from build123d import *

# Parameters (mm, degrees)
SKETCH1_W                    = 49.788
SKETCH1_H                    = 49.788
BOSS_EXTRUDE1_DEPTH          = 3
SKETCH1_3_W                  = 55.788
SKETCH1_3_H                  = 55.788
SKETCH1_3_W_2                = 49.788
SKETCH1_3_H_2                = 49.788
BOSS_EXTRUDE2_DEPTH          = 118
SKETCH2_W                    = 49.788
SKETCH2_H                    = 3
SKETCH2_W_2                  = 43.788
SKETCH2_H_2                  = 38.949
SKETCH2_H_3                  = 26.974
SKETCH2_H_4                  = 16.077
CUT_EXTRUDE1_DEPTH           = 3
FILLET1_R                    = 2
SKETCH3_W                    = 43.788
SKETCH3_H                    = 106
CUT_EXTRUDE2_DEPTH           = 56
FILLET2_R                    = 2
SKETCH4_W                    = 5
SKETCH4_H                    = 3
CUT_EXTRUDE3_DEPTH           = 3
CSK_FOR_M4_SFHCS1_AT_2_COUNT = 2
CSK_FOR_M4_SFHCS1_AT_2_PITCH = 46.834641181
CSK_FOR_M4_SFHCS1_AT_3_COUNT = 2
CSK_FOR_M4_SFHCS1_AT_3_PITCH = 46.834641181
FILLET3_R                    = 1


with BuildPart() as part:
    # Sketch1 → Boss-Extrude1 (new body)
    with BuildSketch(Plane(origin=(0, 0, 0), x_dir=(1, 0, 0), z_dir=(0, 1, 0))):
        Rectangle(SKETCH1_W, SKETCH1_H)
    extrude(amount=BOSS_EXTRUDE1_DEPTH)

    # Sketch1_3 → Boss-Extrude2 (add)
    with BuildSketch(Plane(origin=(0, 0, 0), x_dir=(1, 0, 0), z_dir=(0, 1, 0))):
        Rectangle(SKETCH1_3_W, SKETCH1_3_H)
        Rectangle(SKETCH1_3_W_2, SKETCH1_3_H_2, mode=Mode.SUBTRACT)
    extrude(amount=BOSS_EXTRUDE2_DEPTH)

    # Sketch2 → Cut-Extrude1 (cut)
    with BuildSketch(Plane(origin=(27.894, 0, 0), x_dir=(0, 0, -1), z_dir=(1, 0, 0))):
        with Locations((0, 90.423)):
            Rectangle(SKETCH2_W, SKETCH2_H)
        with Locations((0, 38.474)):
            Rectangle(SKETCH2_W, SKETCH2_H)
        with Locations((0, 64.4485)):
            Rectangle(SKETCH2_W_2, SKETCH2_H_2)
        with Locations((0, 18.487)):
            Rectangle(SKETCH2_W_2, SKETCH2_H_3)
        with Locations((0, 104.9615)):
            Rectangle(SKETCH2_W_2, SKETCH2_H_4)
    extrude(amount=-CUT_EXTRUDE1_DEPTH, mode=Mode.SUBTRACT)

    # Fillet1
    fillet1_edges = [part.edges().sort_by_distance(p)[0] for p in [
        (26.394, 96.923, 21.894),
        (26.394, 113, 21.894),
        (26.394, 113, -21.894),
        (26.394, 96.923, -21.894),
        (26.394, 44.974, 21.894),
        (26.394, 83.923, 21.894),
        (26.394, 83.923, -21.894),
        (26.394, 44.974, -21.894),
        (26.394, 5, 21.894),
        (26.394, 31.974, 21.894),
        (26.394, 31.974, -21.894),
        (26.394, 5, -21.894),
    ]]
    fillet(fillet1_edges, radius=FILLET1_R)

    # Sketch3 → Cut-Extrude2 (cut)
    with BuildSketch(Plane(origin=(0, 0, -27.894), x_dir=(-1, 0, 0), z_dir=(0, 0, -1))):
        with Locations((0, 59)):
            Rectangle(SKETCH3_W, SKETCH3_H)
    extrude(amount=-CUT_EXTRUDE2_DEPTH, mode=Mode.SUBTRACT)

    # Fillet2
    fillet2_edges = [part.edges().sort_by_distance(p)[0] for p in [
        (21.894, 6, -26.394),
        (21.894, 6, 26.394),
        (21.894, 112, -26.394),
        (21.894, 112, 26.394),
        (-21.894, 112, -26.394),
        (-21.894, 112, 26.394),
        (-21.894, 6, -26.394),
        (-21.894, 6, 26.394),
    ]]
    fillet(fillet2_edges, radius=FILLET2_R)

    # Sketch4 → Cut-Extrude3 (cut)
    with BuildSketch(Plane.ZY.offset(27.894)):
        with Locations((0, 90.423)):
            Rectangle(SKETCH4_W, SKETCH4_H)
        with Locations((0, 40.474)):
            Rectangle(SKETCH4_W, SKETCH4_H)
    extrude(amount=-CUT_EXTRUDE3_DEPTH, mode=Mode.SUBTRACT)

    # Sketch7 → CSK for M4 SFHCS1 (revolve, cut)
    with BuildSketch(Plane(origin=(-24.894, 65.538290214, -0.216772751), x_dir=(0, 0, -1), z_dir=(0, 1, 0))):
        Polygon((0, 0), (0, 3), (2.25, 3), (2.25, 2.23), (4.48, 0), align=None)
    csk_for_m4_sfhcs1 = revolve(axis=Axis((-18.544, 65.538290214, -0.216772751), (-1, 0, 0)), mode=Mode.SUBTRACT)

    # CSK for M4 SFHCS1 at 2: CSK for M4 SFHCS1 ×2
    with Locations(*[Vector(0, -0.999997358, -0.002298525) * (i * CSK_FOR_M4_SFHCS1_AT_2_PITCH) for i in range(1, CSK_FOR_M4_SFHCS1_AT_2_COUNT)]):
        add(csk_for_m4_sfhcs1, mode=Mode.SUBTRACT)

    # CSK for M4 SFHCS1 at 3: CSK for M4 SFHCS1 ×2
    with Locations(*[Vector(0, -0.999997358, -0.002298525) * (i * CSK_FOR_M4_SFHCS1_AT_3_PITCH) for i in range(1, CSK_FOR_M4_SFHCS1_AT_3_COUNT)]):
        add(csk_for_m4_sfhcs1, mode=Mode.SUBTRACT)

    # Fillet3
    fillet3_edges = [part.edges().sort_by_distance(p)[0] for p in [
        (24.894, 118, 0),
        (0, 118, -24.894),
        (-24.894, 118, 0),
        (0, 118, 24.894),
        (-27.894, 118, 0),
        (0, 118, 27.894),
        (27.894, 118, 0),
        (0, 118, -27.894),
        (-27.894, 0, 0),
        (-27.894, 59, -27.894),
        (0, 0, 27.894),
        (-27.894, 59, 27.894),
        (27.894, 0, 0),
        (27.894, 59, 27.894),
        (0, 0, -27.894),
        (27.894, 59, -27.894),
    ]]
    fillet(fillet3_edges, radius=FILLET3_R)


solid = part.part
Here's how the part is built. I have some questions about the finished solid (model axes, mm). A direction names the side the tool comes from. Coordinates: 2 decimals unless noted, no trailing zeros. Write each loop counter-clockwise with the first axis right and the second up, starting at its lowest first coordinate (ties: lowest second). Pieces come first, ordered by that corner, then holes. Notation, with made-up numbers: (-29.5, -0.5) - (25.5, -0.5) arc R32 ccw to (25.5, 36.5) - close; hole circle Ø2 at (51, 71). An arc over 180 degrees is marked (long way). Use one line per item in the form item = value.
1) Suppose I cut it at A-A, the plane z = 7. Give the number of separate pieces and of enclosed holes in the cut face, plus the area to 3 significant figures.
Solved:
separate_pieces = 6
enclosed_holes = 0
area = 592 mm2
2) Thinking about a two-plate mould opening in Z: for faces 4 (the flat face through (0, 112, 26)), 5 (the flat face through (-26, 38.974, 0)), 6 (the flat face through (-24, 42, -27.894)), which applies, released by +Z, released by -Z, zero draft, split by the parting line, or undercut?
Solved:
face_4 = zero draft
face_5 = undercut
face_6 = released by -Z
3) On a 3-axis mill with a long thin cutter (end or side, diameter ignored), from which of +Z, -Z, +X, -X, +Y, -Y can I reach the whole of each face in a straight line? I mean faces 1 (the flat face through (26, 88.923, 0)), 2 (the flat face through (0, 6, 26)), 3 (the flat face through (-26, 88.923, 0)). Say none if no direction works.
Solved:
face_1 = +X
face_2 = +Z, -Z
face_3 = +X, -X
4) Suppose I cut it at C-C, the plane y = 105. Write out the boundary of the cut face in (x, z).
Solved:
outline = (-27.89, -26.89) arc R1 ccw to (-26.89, -27.89) - (-21.89, -27.89) - (-21.89, -24.89) - (-24.89, -24.89) - (-24.89, 24.89) - (-21.89, 24.89) - (-21.89, 27.89) - (-26.89, 27.89) arc R1 ccw to (-27.89, 26.89) - close; (21.89, -27.89) - (26.89, -27.89) arc R1 ccw to (27.89, -26.89) - (27.89, -21.89) - (24.89, -21.89) - (24.89, -24.89) - (21.89, -24.89) - close; (21.89, 24.89) - (24.89, 24.89) - (24.89, 21.89) - (27.89, 21.89) - (27.89, 26.89) arc R1 ccw to (26.89, 27.89) - (21.89, 27.89) - close
5) I need wall thicknesses on line 1 (X direction, y = 85.5, z = 25); line 2 (X direction, y = 88.5, z = -20). Which ranges of each line are inside material? Lowest first, please.
Solved:
line_1 = -27.89 to -21.89, 21.89 to 27.89
line_2 = -27.89 to -24.89, 24.89 to 27.89
6) Suppose I cut it at D-D, the plane x = 1. Write out the boundary of the cut face in (y, z).
Solved:
outline = (0, -26.89) arc R1 ccw to (1, -27.89) - (6, -27.89) - (6, -24.89) - (3, -24.89) - (3, 24.89) - (6, 24.89) - (6, 27.89) - (1, 27.89) arc R1 ccw to (0, 26.89) - close; (112, -27.89) - (117, -27.89) arc R1 ccw to (118, -26.89) - (118, -25.89) arc R1 ccw to (117, -24.89) - (112, -24.89) - close; (112, 24.89) - (117, 24.89) arc R1 ccw to (118, 25.89) - (118, 26.89) arc R1 ccw to (117, 27.89) - (112, 27.89) - close
7) Suppose I cut it at B-B, the plane y = 90.5. Write out the boundary of the cut face in (x, z).
Solved:
outline = (-27.89, -26.89) arc R1 ccw to (-26.89, -27.89) - (-21.89, -27.89) - (-21.89, -24.89) - (-24.89, -24.89) - (-24.89, -2.5) - (-27.89, -2.5) - close; (-27.89, 2.5) - (-24.89, 2.5) - (-24.89, 24.89) - (-21.89, 24.89) - (-21.89, 27.89) - (-26.89, 27.89) arc R1 ccw to (-27.89, 26.89) - close; (21.89, -27.89) - (26.89, -27.89) arc R1 ccw to (27.89, -26.89) - (27.89, -24.89) - (21.89, -24.89) - close; (21.89, 24.89) - (27.89, 24.89) - (27.89, 26.89) arc R1 ccw to (26.89, 27.89) - (21.89, 27.89) - close
8) I'm going to push flat-ended pins straight in: P1, Ø10, axis at x = 1.5, z = -1.5, coming from the +Y side; P2, Ø1.5, axis at x = 27, z = 4.5, coming from the -Y side. Where does each tip first touch, or does it pass through?
Solved:
P1 = 3
P2 = 0
